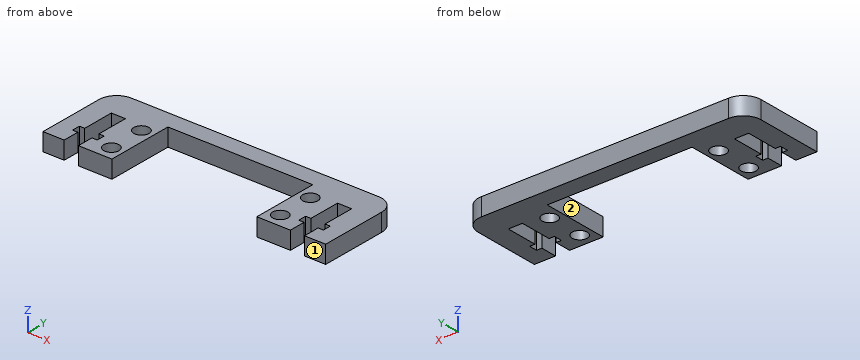
from build123d import *

# Parameters (mm, degrees)
ESQUISSE1_R             = 2.15
BOSS_EXTRU_1_DEPTH      = 5
ENL_V_MAT_EXTRU_2_DEPTH = 30


with BuildPart() as part:
    # Esquisse1 → Boss.-Extru.1 (new body)
    with BuildSketch(Plane.XY):
        with BuildLine():
            Line((-19.5, 0), (0, 0))
            Line((0, 0), (0, 19))
            Line((0, 19), (41, 19))
            Line((41, 19), (41, 0))
            Line((41, 0), (60.5, 0))
            Line((60.5, 0), (60.5, 19))
            ThreePointArc((60.5, 19), (59.035533906, 22.535533906), (55.5, 24))
            Line((55.5, 24), (-14.5, 24))
            ThreePointArc((-14.5, 24), (-18.035533906, 22.535533906), (-19.5, 19))
            Line((-19.5, 19), (-19.5, 0))
        make_face()
        with Locations((44.4, 14.1)):
            Circle(ESQUISSE1_R, mode=Mode.SUBTRACT)
        with Locations((44.4, 3.9)):
            Circle(ESQUISSE1_R, mode=Mode.SUBTRACT)
        with Locations((-3.4, 14.1)):
            Circle(ESQUISSE1_R, mode=Mode.SUBTRACT)
        with Locations((-3.4, 3.9)):
            Circle(ESQUISSE1_R, mode=Mode.SUBTRACT)
    extrude(amount=BOSS_EXTRU_1_DEPTH)

    # Esquisse3 → Enlèv. mat.-Extru.2 (cut)
    with BuildSketch(Plane.XY.offset(5)):
        Polygon((-9.5, 3.002605055), (-9.5, 4.625752713), (-8, 4.625752713), (-8, 6.971671519), (-9.5, 6.971671519), (-9.5, 16), (-13.5, 16), (-13.5, 6.971671519), (-15, 6.971671519), (-15, 4.625752713), (-13.5, 4.625752713), (-13.5, 3.002605055), (-13.5, 0), (-9.5, 0), align=None)
        Polygon((54.5, 0), (50.5, 0), (50.5, 3.002605055), (50.5, 4.625752713), (49, 4.625752713), (49, 6.971671519), (50.5, 6.971671519), (50.5, 16), (54.5, 16), (54.5, 6.971671519), (56, 6.971671519), (56, 4.625752713), (54.5, 4.625752713), (54.5, 3.002605055), align=None)
    extrude(amount=-ENL_V_MAT_EXTRU_2_DEPTH, mode=Mode.SUBTRACT)


solid = part.part
Part model, mm, in its own coordinate system. Face numbers are marked on the shaded views. A direction names the side the tool comes from. Round coordinates to 2 decimals unless told otherwise and drop trailing zeros. Write each loop counter-clockwise with the first axis right and the second up, starting at its lowest first coordinate (ties: lowest second). Pieces come first, ordered by that corner, then holes. Notation, with made-up numbers: (42.5, 82) - (83.5, 82) arc R20 ccw to (83.5, 87) - close; hole circle Ø7 at (82.5, 67.5). An arc over 180 degrees is marked (long way). Use CSV: the item, a comma, the result in double quotes.
Item 1: Slice it at C-C, the plane z = 2.25. Count the separate pieces of the cut face and the enclosed holes in it, then the cut area to 3 significant figures.
Results list:
separate pieces,"1"
enclosed holes,"4"
area,"930 mm²"
Item 2: Slice it at D-D, the plane x = 13.5. Write the cut outline in (y, z).
Results list:
outline,"(19, 0) - (24, 0) - (24, 5) - (19, 5) - close"
Item 3: Tool access for the marked faces 1 and 2: list every direction of +Z, -Z, +X, -X, +Y, -Y with a clear straight run to the whole face (end or side of a thin tool).
Results list:
face 1,"+Z, -Z, +X, -X, -Y"
face 2,"+Z, -Z, -Y"
Item 4: Slice it at B-B, the plane x = -3.4. Write the cut outline in (y, z).
Results list:
outline,"(0, 0) - (1.75, 0) - (1.75, 5) - (0, 5) - close; (6.05, 0) - (11.95, 0) - (11.95, 5) - (6.05, 5) - close; (16.25, 0) - (24, 0) - (24, 5) - (16.25, 5) - close"
Item 5: Wall check: L1, parallel to Y at x = 44.4, z = 1.1; L2, parallel to X at y = 1.5, z = 0.5; L3, parallel to X at y = 6.5, z = 3.7. Give the ranges that are in metal, low to high.
Results list:
L1,"y = 0 to 1.75, 6.05 to 11.95, 16.25 to 24"
L2,"x = -19.5 to -13.5, -9.5 to 0, 41 to 50.5, 54.5 to 60.5"
L3,"x = -19.5 to -15, -8 to 0, 41 to 49, 56 to 60.5"
Item 6: Slice it at A-A, the plane y = 14.1. Write the cut outline in (x, z), then the cut area to 3 significant figures.
Results list:
outline,"(-19.5, 0) - (-13.5, 0) - (-13.5, 5) - (-19.5, 5) - close; (-9.5, 0) - (-5.55, 0) - (-5.55, 5) - (-9.5, 5) - close; (-1.25, 0) - (0, 0) - (0, 5) - (-1.25, 5) - close; (41, 0) - (42.25, 0) - (42.25, 5) - (41, 5) - close; (46.55, 0) - (50.5, 0) - (50.5, 5) - (46.55, 5) - close; (54.5, 0) - (60.5, 0) - (60.5, 5) - (54.5, 5) - close"
area,"112 mm²"
Item 7: Flat gauge pins, fed straight in: P1, Ø1.5, axis at x = 51.5, z = 1.5, coming from the -Y side; P2, Ø1.5, axis at x = 15, z = 1.5, coming from the -Y side. Where does each tip first touch, or does it go through?
Results list:
P1,"stops at y = 16"
P2,"stops at y = 19"
